Read the model definition and answer for the solid it produces. Units are mm, in the model's axes. A direction names the side the tool comes from. Give positions to 0.01 mm unless a question says otherwise; leave off trailing zeros. Order: outer loops, then holes, each group sorted by start corner. A loop starts at its lowest first (then second) coordinate and runs counter-clockwise, first axis right, second up. Notation, with made-up numbers: (64.25, 87) - (117.25, 87) arc R13 cw to (117.25, 112) - close; hole circle Ø4 at (15, -34). An arc over 180 degrees is marked (long way). One line per item, written item: value. Start each with the question number.
```python
from build123d import *

# Parameters (mm, degrees)
SKETCH1_W               = 14
SKETCH1_H               = 35
BOSS_EXTRUDE1_DEPTH     = 16.5
CUT_EXTRUDE3_DEPTH      = 37.989863476
CUT_EXTRUDE3_DEPTH_BACK = 37.989863476
SKETCH3_OUTSIDE_W       = 24.23
SKETCH3_OUTSIDE_H       = 45.23
SKETCH3_OUTSIDE_W_2     = 14
SKETCH3_OUTSIDE_H_2     = 35
SKETCH3_OUTSIDE_W_3     = 12
SKETCH3_OUTSIDE_H_3     = 33
CUT_EXTRUDE4_DEPTH      = 37.989863476
CUT_EXTRUDE4_DEPTH_BACK = 40.5
SKETCH4_R               = 3.6
SKETCH5_R               = 1.25
CUT_EXTRUDE6_DEPTH      = 1


with BuildPart() as part:
    # Sketch1 → Boss-Extrude1 (new body)
    with BuildSketch(Plane.XY):
        with Locations((7, 12.5)):
            Rectangle(SKETCH1_W, SKETCH1_H)
    extrude(amount=BOSS_EXTRUDE1_DEPTH)

    # Sketch3 outside → Cut-Extrude3 (cut, two sides: drawn at the far end of the back side and taken through both)
    # profile 1 of 2: a face of its own
    with BuildSketch(Plane.XY.offset(-CUT_EXTRUDE3_DEPTH_BACK)):
        with Locations((7, 12.5)):
            Rectangle(SKETCH3_OUTSIDE_W, SKETCH3_OUTSIDE_H)
        with Locations((7, 12.5)):
            Rectangle(SKETCH3_OUTSIDE_W_2, SKETCH3_OUTSIDE_H_2, mode=Mode.SUBTRACT)
    # profile 2 of 2: a face of its own
    with BuildSketch(Plane.XY.offset(-CUT_EXTRUDE3_DEPTH_BACK)):
        with Locations((7, 12.5)):
            Rectangle(SKETCH3_OUTSIDE_W_3, SKETCH3_OUTSIDE_H_3)
    extrude(amount=CUT_EXTRUDE3_DEPTH + CUT_EXTRUDE3_DEPTH_BACK, mode=Mode.SUBTRACT)

    # Sketch4 → Cut-Extrude4 (cut, two sides: drawn at the far end of the back side and taken through both)
    with BuildSketch(Plane(origin=(0, 0, 0), x_dir=(1, 0, 0), z_dir=(0, 1, 0)).offset(-CUT_EXTRUDE4_DEPTH_BACK)):
        with Locations((7, -8.25)):
            Circle(SKETCH4_R)
    extrude(amount=CUT_EXTRUDE4_DEPTH + CUT_EXTRUDE4_DEPTH_BACK, mode=Mode.SUBTRACT)

    # Sketch5 → Cut-Extrude6 (cut)
    with BuildSketch(Plane(origin=(0, 0, 0), x_dir=(0, 0, -1), z_dir=(1, 0, 0))):
        with Locations(Location((-4.939666778, 25, 0), (0, 0, 270))):
            Circle(SKETCH5_R)
        with Locations(Location((-12.939666778, 5, 0), (0, 0, 270))):
            Circle(SKETCH5_R)
    extrude(amount=CUT_EXTRUDE6_DEPTH, mode=Mode.SUBTRACT)


solid = part.part
```
1) Section B-B on x = 7 is taken. Write down the section's boundary in (y, z), plus the area to 3 significant figures.
2) Section D-D on y = 25 is taken. Write down the section's boundary in (x, z).
3) For faces 1 (the cylindrical face through (0.493, 23.845, 5.418)), 2 (the flat face through (0.7, 13.9, 16.5)), 3 (the flat face through (1, 12, 8)), determine the directions among +Z, -Z, +X, -X, +Y, -Y from which every point of the face is accessible in a straight line to the end or side of a thin tool.
4) Find the intervals of material crossed by probe 1 along X at (y, z) = (2, 13.75); probe 2 along Y at (x, z) = (4.25, 2.25); probe 3 along Z at (x, y) = (7, -4.2), in increasing order. Write a range as from..to.
5) The mould has two halves that part along X. Classify faces 4 (the flat face through (14, 12, 8)), 5 (the flat face through (7, 29, 4)), 6 (the flat face through (3.79, 30, 6.3)): +X half, -X half, draft (parallel to the pull), parting line (faces both ways), or undercut.
6) Section A-A on y = 12 is taken. Write down the section's boundary in (x, z), plus the area to 3 significant figures.
7) Section C-C on z = 11 is taken. Write down the section's boundary in (x, y), plus the area to 3 significant figures.
8) This flat-tipped pin is pushed along its axis until it touches: pin 1 (3 mm diameter, centred on y = 9, z = 11, fed in from -X). Where does it stop, or does it pass through?
Solved:
1. outline: (-5, 0) - (-4, 0) - (-4, 4.65) - (-5, 4.65) - close; (-5, 11.85) - (-4, 11.85) - (-4, 16.5) - (-5, 16.5) - close; (29, 0) - (30, 0) - (30, 4.65) - (29, 4.65) - close; (29, 11.85) - (30, 11.85) - (30, 16.5) - (29, 16.5) - close
1. area: 18.6 mm2
2. outline: (0, 0) - (1, 0) - (1, 3.69) - (0, 3.69) - close; (0, 6.19) - (1, 6.19) - (1, 16.5) - (0, 16.5) - close; (13, 0) - (14, 0) - (14, 16.5) - (13, 16.5) - close
3. face 1: -X
3. face 2: +Z, +X, -X, +Y, -Y
3. face 3: +Z, -Z
4. probe 1: x = 0..1, 13..14
4. probe 2: y = -5..-4, 29..30
4. probe 3: z = 0..4.65, 11.85..16.5
5. face 4: +X half
5. face 5: undercut
5. face 6: draft
6. outline: (0, 0) - (1, 0) - (1, 16.5) - (0, 16.5) - close; (13, 0) - (14, 0) - (14, 16.5) - (13, 16.5) - close
6. area: 33.0 mm2
7. outline: (0, -5) - (4.68, -5) - (4.68, -4) - (1, -4) - (1, 29) - (4.68, 29) - (4.68, 30) - (0, 30) - close; (9.32, -5) - (14, -5) - (14, 30) - (9.32, 30) - (9.32, 29) - (13, 29) - (13, -4) - (9.32, -4) - close
7. area: 84.7 mm2
8. pin 1: stops at x = 0
